```python
from build123d import *

# Parameters (mm, degrees)
SKETCH1_W           = 82.55
SKETCH1_H           = 44.45
BOSS_EXTRUDE1_DEPTH = 6.35
SKETCH2_W           = 5.588
SKETCH2_H           = 18.288
BOSS_EXTRUDE2_DEPTH = 6.35
SKETCH5_W           = 18.288
SKETCH5_H           = 5.588
BOSS_EXTRUDE3_DEPTH = 6.35
SKETCH3_W           = 5.588
SKETCH3_H           = 18.288
CUT_EXTRUDE1_DEPTH  = 97.739994025
SKETCH6_R           = 1.524
CUT_EXTRUDE2_DEPTH  = 97.739994025
SKETCH7_W           = 12.065
SKETCH7_H           = 10.16
CUT_EXTRUDE4_DEPTH  = 97.739994025


with BuildPart() as part:
    # Sketch1 → Boss-Extrude1 (new body)
    with BuildSketch(Plane.XY):
        with Locations((41.275, 22.225)):
            Rectangle(SKETCH1_W, SKETCH1_H)
    extrude(amount=BOSS_EXTRUDE1_DEPTH)

    # Sketch2 → Boss-Extrude2 (add)
    with BuildSketch(Plane.XY.offset(6.35)):
        with Locations((-2.794, 22.225)):
            Rectangle(SKETCH2_W, SKETCH2_H)
    extrude(amount=-BOSS_EXTRUDE2_DEPTH)

    # Sketch5 → Boss-Extrude3 (add)
    with BuildSketch(Plane.XY.offset(6.35)):
        with Locations((38.481, 47.244)):
            Rectangle(SKETCH5_W, SKETCH5_H)
        with Locations((38.481, -2.794)):
            Rectangle(SKETCH5_W, SKETCH5_H)
    extrude(amount=-BOSS_EXTRUDE3_DEPTH)

    # Sketch3 → Cut-Extrude1 (cut, through all)
    with BuildSketch(Plane.XY.offset(6.35)):
        with Locations((79.756, 22.225)):
            Rectangle(SKETCH3_W, SKETCH3_H)
    extrude(amount=-CUT_EXTRUDE1_DEPTH, mode=Mode.SUBTRACT)

    # Sketch6 → Cut-Extrude2 (cut, through all)
    with BuildSketch(Plane.XY.offset(6.35)):
        with Locations((-2.794, 22.225)):
            Circle(SKETCH6_R)
        with Locations((38.481, -2.794)):
            Circle(SKETCH6_R)
        with Locations((38.481, 47.244)):
            Circle(SKETCH6_R)
        Polygon((67.437, 23.8125), (70.612, 23.8125), (70.612, 26.035), (73.787, 26.035), (73.787, 23.8125), (76.962, 23.8125), (76.962, 20.6375), (73.787, 20.6375), (73.787, 18.415), (70.612, 18.415), (70.612, 20.6375), (67.437, 20.6375), align=None)
    extrude(amount=-CUT_EXTRUDE2_DEPTH, mode=Mode.SUBTRACT)

    # Sketch7 → Cut-Extrude4 (cut, through all)
    with BuildSketch(Plane.XY):
        with Locations((27.2415, 16.51)):
            Rectangle(SKETCH7_W, SKETCH7_H)
    extrude(amount=CUT_EXTRUDE4_DEPTH, mode=Mode.SUBTRACT)


solid = part.part
```
Geometry: final body of the model. Coordinates: model frame, mm. A direction names the side the tool comes from. Coordinates: 2 decimals unless noted, no trailing zeros. Loops run counter-clockwise (first coordinate to the right, second up) from the corner with the lowest first, then second, coordinate; pieces in that order, holes last. Notation, with made-up numbers: M 60,-8.5 L 110,-8.5 A26 cw 110,14.5 Z; hole C 1.5,-1.75 d5. An arc over 180 degrees is marked long. Put each result on its own line as item: value.
(1) Access query for faces 1 (the face through (70.612, 20, 3)), 2 (the face through (65, 44.45, 3)), 3 (the face through (76.962, 17, 3)), 4 (the face through (29.337, -3, 3)). Directions: +Z, -Z, +X, -X, +Y, -Y. A direction counts if a zero-diameter tool reaches every point of the face in a straight line with its end or side. Return the directions, or none.
Answer sheet:
face 1: +Z, -Z
face 2: +Z, -Z, +X, +Y
face 3: +Z, -Z, +X
face 4: +Z, -Z, -X, -Y
(2) Material intervals for probe 1 along X at (y, z) = (19, 4.25); probe 2 along Y at (x, z) = (70.5, 5.5); probe 3 along Y at (x, z) = (27.5, 5.5), sorted ascending.
Answer sheet:
probe 1: x = -5.59 to 21.21, 33.27 to 70.61, 73.79 to 76.96
probe 2: y = 0 to 20.64, 23.81 to 44.45
probe 3: y = 0 to 11.43, 21.59 to 44.45
(3) Cut plane D-D on x = 5. Return the cut outline in (y, z), then the cut area to 3 significant figures.
Answer sheet:
outline: M 0,0 L 44.45,0 L 44.45,6.35 L 0,6.35 Z
area: 282 mm^2
(4) Cut plane A-A on x = 75. Return the cut outline in (y, z).
Answer sheet:
outline: M 0,0 L 20.64,0 L 20.64,6.35 L 0,6.35 Z; M 23.81,0 L 44.45,0 L 44.45,6.35 L 23.81,6.35 Z
(5) First-contact query: pin 1 (2.5 mm diameter, centred on x = 68.5, z = 3, fed in from +Y); pin 2 (1.6 mm diameter, centred on x = 72.5, z = 4.5, fed in from -Y); pin 3 (1.1 mm diameter, centred on y = 19, z = 2, fed in from +X). Flat tips, straight axial feed; report the tip coordinate or a pass-through.
Answer sheet:
pin 1: stops at y = 44.45
pin 2: stops at y = 0
pin 3: stops at x = 76.96
(6) Cut plane C-C on y = 6.5. Return the cut outline in (x, z).
Answer sheet:
outline: M 0,0 L 82.55,0 L 82.55,6.35 L 0,6.35 Z
(7) Draft query along Y for faces 5 (the face through (38, -5.588, 3)), 6 (the face through (82.55, 6, 3)), 7 (the face through (75, 23.812, 3)). Return one class per face: pulls with the +Y half, pulls with the -Y half, needs draft (parallel to the pull), parting line crosses it, or undercut.
Answer sheet:
face 5: pulls with the -Y half
face 6: needs draft
face 7: undercut
(8) Cut plane B-B on x = 39. Return the cut outline in (y, z), then the cut area to 3 significant figures.
Answer sheet:
outline: M -5.59,0 L -4.23,0 L -4.23,6.35 L -5.59,6.35 Z; M -1.36,0 L 45.81,0 L 45.81,6.35 L -1.36,6.35 Z; M 48.68,0 L 50.04,0 L 50.04,6.35 L 48.68,6.35 Z
area: 317 mm^2
